For this review, take the finished solid that the model builds, in its own axes (mm). A direction names the side the tool comes from. Coordinates: 2 decimals unless noted, no trailing zeros. Order: outer loops, then holes, each group sorted by start corner. A loop starts at its lowest first (then second) coordinate and runs counter-clockwise, first axis right, second up. Notation, with made-up numbers: M -34,43.25 L -26,43.25 A13 ccw -26,54.25 Z; hole C -5.5,-16.5 d6. An arc over 180 degrees is marked long. Use CSV: the item, a comma, the result in double quotes.
```python
from build123d import *

# Parameters (mm, degrees)
CUT_EXTRUDE1_START = 11.896721
SKETCH3_R          = 4.445
CUT_EXTRUDE1_DEPTH = 2.54
SKETCH4_R          = 3.175
CUT_EXTRUDE2_DEPTH = 7.62
CUT_EXTRUDE3_START = 11.896721
SKETCH5_R          = 4.445
CUT_EXTRUDE3_DEPTH = 7.62
SKETCH6_R          = 3.175
CUT_EXTRUDE4_DEPTH = 7.62


with BuildPart() as part:
    # Sketch2 → Revolve2 (revolve)
    with BuildSketch(Plane.XY):
        with BuildLine():
            Line((0, 12.7), (0, -12.7))
            ThreePointArc((0, -12.7), (12.7, 0), (0, 12.7))
        make_face()
    revolve(axis=Axis((0, 0, 0), (0, 1, 0)))

    # Sketch3 → Cut-Extrude1 (cut)
    with BuildSketch(Plane.XY.offset(CUT_EXTRUDE1_START)):
        Circle(SKETCH3_R)
    cut_extrude1 = extrude(amount=CUT_EXTRUDE1_DEPTH, mode=Mode.SUBTRACT)

    # Sketch4 → Cut-Extrude2 (cut)
    with BuildSketch(Plane.XY.offset(11.896721187)):
        Circle(SKETCH4_R)
    cut_extrude2 = extrude(amount=-CUT_EXTRUDE2_DEPTH, mode=Mode.SUBTRACT)

    # Mirror1: Cut-Extrude1, Cut-Extrude2 across plane
    add(cut_extrude1.mirror(Plane.XY), mode=Mode.SUBTRACT)
    add(cut_extrude2.mirror(Plane.XY), mode=Mode.SUBTRACT)

    # Sketch5 → Cut-Extrude3 (cut)
    with BuildSketch(Plane(origin=(0, 0, 0), x_dir=(1, 0, 0), z_dir=(0, 1, 0)).offset(CUT_EXTRUDE3_START)):
        Circle(SKETCH5_R)
    extrude(amount=CUT_EXTRUDE3_DEPTH, mode=Mode.SUBTRACT)

    # Sketch6 → Cut-Extrude4 (cut)
    with BuildSketch(Plane(origin=(0, 11.896721187, 0), x_dir=(1, 0, 0), z_dir=(0, 1, 0))):
        with Locations(Location((0, 0, 0), (0, 0, 270))):
            Circle(SKETCH6_R)
    extrude(amount=-CUT_EXTRUDE4_DEPTH, mode=Mode.SUBTRACT)


solid = part.part
```
Item 1: For faces 5 (the face through (0, 0, 4.277)), 6 (the face through (-1.93, 8.14, -2.52)), 7 (the face through (-0.69, -3.1, -8.14)), list the 3-axis set-ups (+Z, -Z, +X, -X, +Y, -Y) from which the entire face can be reached by the end or side of a thin tool; tool diameter is ignored.
Solutions:
face 5,"+Z"
face 6,"+Y"
face 7,"-Z"
Item 2: To check wall thickness, follow line 1 along X through (y, z) = (2, 9.25); line 2 along X through (y, z) = (9.25, -2.5); line 3 along Y through (x, z) = (-2.5, 8.5). State the ranges of each line that lie inside material, in increasing order. Write a range as [from, to].
Solutions:
line 1,"[-8.47, -2.47], [2.47, 8.47]"
line 2,"[-8.34, -1.96], [1.96, 8.34]"
line 3,"[-9.1, -1.96], [1.96, 9.1]"
Item 3: Add section A-A on y = 0. State the section outline as (x, z) points (3 decimals), and give its area (3 significant figures).
Solutions:
outline,"M -4.445,-11.897 L -3.175,-11.897 L -3.175,-4.277 L 3.175,-4.277 L 3.175,-11.897 L 4.445,-11.897 A12.7 ccw 4.445,11.897 L 3.175,11.897 L 3.175,4.277 L -3.175,4.277 L -3.175,11.897 L -4.445,11.897 A12.7 ccw Z"
area,"400 mm^2"
Item 4: Add section B-B on z = 0. State the section outline as (x, y) points (3 decimals).
Solutions:
outline,"M -4.445,11.897 A12.7 ccw long 4.445,11.897 L 3.175,11.897 L 3.175,4.277 L -3.175,4.277 L -3.175,11.897 Z"
Item 5: Add section C-C on z = -5.5. State the section outline as (x, y) points (3 decimals), and give its area (3 significant figures).
Solutions:
outline,"C 0,0 d22.895; hole C 0,0 d6.35"
area,"380 mm^2"
Item 6: Add section D-D on x = -5.25. State the section outline as (y, z) points, and give its area (3 significant figures).
Solutions:
outline,"C 0,0 d23.13"
area,"420 mm^2"
Item 7: Clearance check with flat-ended pins moving along their axes: pin 1 Ø4 at (y, z) = (0, 3) entering from +X; pin 2 Ø3 at (x, z) = (-5.5, 0.5) entering from -Y; pin 3 Ø1.5 at (y, z) = (6, -6.5) entering from +X (3 decimals). State where each tip first meets the part, or that it passes through.
Solutions:
pin 1,"x = 12.66"
pin 2,"y = -12.05"
pin 3,"x = 9.785"
Item 8: Draft analysis for pull direction Z (two halves, no side actions). For faces 1 (the face through (2, -3, -11.897)), 2 (the face through (2, -3, 11.897)), 3 (the face through (-0.69, -3.1, 8.14)), 4 (the face through (0, 4.277, 0)), state which applies: released by +Z, released by -Z, zero draft, split by the parting line, or undercut.
Solutions:
face 1,"released by -Z"
face 2,"released by +Z"
face 3,"zero draft"
face 4,"undercut"
